Geometry check sheet. Reference: the model listing, model coordinates, mm. A direction names the side the tool comes from. Coordinates: 2 decimals unless noted, no trailing zeros. Loops run counter-clockwise (first coordinate to the right, second up) from the corner with the lowest first, then second, coordinate; pieces in that order, holes last.
from build123d import *

# Parameters (mm, degrees)
PAD059_DEPTH         = 10
POCKET157_DEPTH      = 10.001
POCKET157_DEPTH_BACK = 10.001
SKETCH188_R          = 2.1
HOLE055_DEPTH        = 25
HOLE055_TIPS_R       = 2.1
SKETCH_W             = 10
SKETCH_H             = 5
POCKET_DEPTH         = 3
CHAMFER001_SIZE      = 0.4


with BuildPart() as part:
    # Sketch189 → Pad059 (new body, symmetric)
    with BuildSketch(Plane.XZ):
        with BuildLine():
            Line((-10, 0), (-10, 30))
            ThreePointArc((-9.548077, 32.972243), (-9.886374, 31.503202), (-10, 30))
            Line((-1.1, 28.094744), (-9.548077, 32.972243))
            ThreePointArc((-1.1, 28.094744), (1.905256, 28.9), (1.1, 31.905256))
            Line((-7.348077, 36.782755), (1.1, 31.905256))
            ThreePointArc((8.660254, 35), (1.1068, 39.938561), (-7.348077, 36.782755))
            Line((8.660254, 35), (10, 32.679492))
            Line((10, 0), (10, 32.679492))
            Line((10, 0), (3, 0))
            Line((3, 0), (1.845299, -2))
            Line((1.845299, -2), (-3, -2))
            Line((-3, -2), (-3, 0))
            Line((-10, 0), (-3, 0))
        make_face()
    extrude(amount=PAD059_DEPTH, both=True)

    # Sketch190 → Pocket157 (cut, two sides)
    with BuildSketch(Plane.YZ) as pocket157_sk:
        with BuildLine():
            Line((6, 18.5), (6, 40))
            Line((6, 40), (-6, 40))
            Line((-6, 40), (-6, 18.5))
            ThreePointArc((-8, 14.027864), (-6.522774, 16.05051), (-6, 18.5))
            ThreePointArc((-8, 14.027864), (-9.477226, 12.005218), (-10, 9.555728))
            Line((-10, 9.555728), (-10, 3))
            Line((-10, 3), (-11, 3))
            Line((-11, 3), (-11, 41))
            Line((-11, 41), (11, 41))
            Line((11, 3), (11, 41))
            Line((10, 3), (11, 3))
            Line((10, 9.555728), (10, 3))
            ThreePointArc((10, 9.555728), (9.477226, 12.005218), (8, 14.027864))
            ThreePointArc((6, 18.5), (6.522774, 16.05051), (8, 14.027864))
        make_face()
    extrude(amount=-POCKET157_DEPTH, mode=Mode.SUBTRACT)
    extrude(pocket157_sk.sketch, amount=POCKET157_DEPTH_BACK, mode=Mode.SUBTRACT)

    # Sketch188 → Hole055 (cut)
    with BuildSketch(Plane(origin=(0, 0, -2), x_dir=(-1, 0, 0), z_dir=(0, 0, -1))):
        Circle(SKETCH188_R)
    extrude(amount=-HOLE055_DEPTH, mode=Mode.SUBTRACT)

    # Hole055 tips → Hole055 tip 1 section 0
    with BuildSketch(Plane(origin=(0, 0, 23), x_dir=(-1, 0, 0), z_dir=(0, 0, -1)), mode=Mode.PRIVATE) as hole055_tip_1_s0:
        Circle(HOLE055_TIPS_R)
    loft([hole055_tip_1_s0.sketch, Vertex(0, 0, 24.261807)], mode=Mode.SUBTRACT)

    # Sketch → Pocket (cut, symmetric)
    with BuildSketch(Plane.YZ):
        with Locations((0, -2.5)):
            Rectangle(SKETCH_W, SKETCH_H)
    extrude(amount=POCKET_DEPTH, both=True, mode=Mode.SUBTRACT)

    # Chamfer001
    chamfer001_edges = [part.edges().sort_by_distance(p)[0] for p in [
        (10, 6, 25.589746),
        (10, 6.522774, 16.05051),
        (10, 9.477226, 12.005218),
        (10, 10, 6.277864),
        (10, 10, 1.5),
        (10, 0, 0),
        (10, -10, 6.277864),
        (10, -9.477226, 12.005218),
        (10, -10, 1.5),
        (10, -6.522774, 16.05051),
        (10, -6, 25.589746),
        (-10, 0, 0),
        (-10, 10, 1.5),
        (-10, 10, 6.277864),
        (-10, 9.477226, 12.005218),
        (-10, 6.522774, 16.05051),
        (-10, 6, 24.25),
        (-9.886374, 6, 31.503202),
        (-9.886374, -6, 31.503202),
        (-10, -6, 24.25),
        (-10, -6.522774, 16.05051),
        (-10, -9.477226, 12.005218),
        (-10, -10, 6.277864),
        (-10, -10, 1.5),
        (5, 6, 38.660254),
        (9.330127, 6, 33.839746),
        (-4.010763, 6, 39.160446),
        (-4.010763, -6, 39.160446),
        (5, -6, 38.660254),
        (9.330127, -6, 33.839746),
        (-7.348077, 0, 36.782755),
        (-9.548077, 0, 32.972243),
        (-3.124038, 6, 34.344006),
        (1.905256, 6, 28.9),
        (-5.324038, 6, 30.533494),
        (-3.124038, -6, 34.344006),
        (1.905256, -6, 28.9),
        (-5.324038, -6, 30.533494),
    ]]
    chamfer(chamfer001_edges, length=CHAMFER001_SIZE)


with BuildPart() as part_1:
    # Body022039 placement: moved
    add(part.part.moved(Location((-113, -113, -52))))


solid = part_1.part
1) Access from +Z, -Z, +X, -X, +Y, -Y to the whole of each face (thin tool, end or side, straight path). Record for faces 1 (the flat face through (-116, -106, -53)), 2 (the flat face through (-118.306, -107.203, -21.705)), 3 (the flat face through (-113, -119, -25)), 4 (the conical face through (-111.856, -107.114, -12.354)), 5 (the cylindrical face through (-113.969, -114.863, -40.661)).
Data:
face 1: -Z, -X, +Y, -Y
face 2: +Y
face 3: +Z, +X, -X, -Y
face 4: +Z, +Y
face 5: -Z
2) Section check B-B on z = -27. Record the cut outline in (x, y).
Data:
outline: (-123, -118.6) - (-122.6, -119) - (-103.4, -119) - (-103, -118.6) - (-103, -107.4) - (-103.4, -107) - (-122.6, -107) - (-123, -107.4) - close
3) Section check A-A on y = -110. Record the cut outline in (x, z).
Data:
outline: (-123, -51.6) - (-122.6, -52) - (-103.4, -52) - (-103, -51.6) - (-103, -19.32) - (-104.34, -17) arc R10 ccw to (-120.07, -14.93) - (-120, -15.42) - (-111.9, -20.09) arc R2.2 cw to (-114.1, -23.91) - (-122.2, -19.23) - (-122.66, -19.41) arc R10 ccw to (-123, -22) - close
4) Material ranges on probe 1 along Y at (x, z) = (-105.5, -19.5); probe 2 along Y at (x, z) = (-113, -37); probe 3 along Y at (x, z) = (-113, -46.75), recorded low to high.
Data:
probe 1: y = -119 to -107
probe 2: y = -120.13 to -115.1, -110.9 to -105.87
probe 3: y = -123 to -115.1, -110.9 to -103
5) Depth check by flat-ended pin: pin 1 (9.5 mm diameter, centred on x = -112, z = -27.5, fed in from -Y); pin 2 (2 mm diameter, centred on y = -120.5, z = -53.5, fed in from -X); pin 3 (10 mm diameter, centred on x = -110, z = -19.5, fed in from +Y). Enter the tip coordinate at first touch or a pass-through.
Data:
pin 1: stops at y = -119
pin 2: stops at x = -116
pin 3: stops at y = -107
6) Mould release check, pull along Z, two halves, no side actions. Record for faces 6 (the flat face through (-114, -106, -54)), 7 (the flat face through (-115.91, -118.8, -17.55)), 8 (the flat face through (-103.83, -118.8, -18.28)): +Z half, -Z half, draft (parallel to the pull), parting line (faces both ways), or undercut.
Data:
face 6: -Z half
face 7: undercut
face 8: +Z half
